from build123d import *

# Parameters (mm, degrees)
SKETCH_1_R               = 23.25
SKETCH_1_R_2             = 9
EXTRUDE_1_DEPTH          = 10
SKETCH_2_R               = 5
EXTRUDE_2_DEPTH          = 6
PATTERN_CIRCULAR_1_COUNT = 8
SKETCH_4_R               = 23.5
SKETCH_4_R_2             = 9
EXTRUDE_3_DEPTH          = 8.5


with BuildPart() as part:
    # 草图1 → 凸台-拉伸1 (new, symmetric)
    with BuildSketch(Plane(origin=(0, 0, 0), x_dir=(1, 0, 0), z_dir=(0, 1, 0))):
        with Locations(Location((0, 0, 0), (0, 0, 270))):
            Circle(SKETCH_1_R)
        with Locations(Location((0, 0, 0), (0, 0, 270))):
            Circle(SKETCH_1_R_2, mode=Mode.SUBTRACT)
    extrude(amount=EXTRUDE_1_DEPTH, both=True)

    # 草图2 → 凸台-拉伸2 (add)
    with BuildSketch(Plane(origin=(0, 10, 0), x_dir=(1, 0, 0), z_dir=(0, 1, 0))):
        with Locations(Location((16.25, 0, 0), (0, 0, 270))):
            Circle(SKETCH_2_R)
    extrude_2 = extrude(amount=EXTRUDE_2_DEPTH)

    # 阵列(圆周)1: 凸台-拉伸2 ×8 about axis
    pattern_circular_1_axis = Axis((0, 0, 0), (0, 1, 0))
    for i in range(1, PATTERN_CIRCULAR_1_COUNT):
        add(extrude_2.rotate(pattern_circular_1_axis, i * 360 / PATTERN_CIRCULAR_1_COUNT))

    # 草图4 → 凸台-拉伸3 (add, symmetric)
    with BuildSketch(Plane(origin=(0, 0, 0), x_dir=(1, 0, 0), z_dir=(0, 1, 0))):
        with Locations(Location((0, 0, 0), (0, 0, 270))):
            Circle(SKETCH_4_R)
        with Locations(Location((0, 0, 0), (0, 0, 270))):
            Circle(SKETCH_4_R_2, mode=Mode.SUBTRACT)
    extrude(amount=EXTRUDE_3_DEPTH, both=True)


solid = part.part
Geometry check sheet. Reference: the model listing, model coordinates, mm. A direction names the side the tool comes from. Give positions to 0.01 mm unless a question says otherwise; leave off trailing zeros. Loops run counter-clockwise (first coordinate to the right, second up) from the corner with the lowest first, then second, coordinate; pieces in that order, holes last.
(1) Section check B-B on x = 0. Record the cut outline in (y, z).
From the geometry:
outline: (-10, -23.25) - (-8.5, -23.25) - (-8.5, -23.5) - (8.5, -23.5) - (8.5, -23.25) - (10, -23.25) - (10, -21.25) - (16, -21.25) - (16, -11.25) - (10, -11.25) - (10, -9) - (-10, -9) - close; (-10, 9) - (10, 9) - (10, 11.25) - (16, 11.25) - (16, 21.25) - (10, 21.25) - (10, 23.25) - (8.5, 23.25) - (8.5, 23.5) - (-8.5, 23.5) - (-8.5, 23.25) - (-10, 23.25) - close
(2) Depth check by flat-ended pin: pin 1 Ø4 at (x, y) = (2.5, -1) entering from +Z; pin 2 Ø6 at (x, y) = (-18, 0.5) entering from -Z; pin 3 Ø1.5 at (y, z) = (-7, 16) entering from +X; pin 4 Ø11 at (x, z) = (0, 0) entering from +Y. Enter the tip coordinate at first touch or a pass-through.
From the geometry:
pin 1: stops at z = 23.49
pin 2: stops at z = -18.09
pin 3: stops at x = 17.88
pin 4: passes through
(3) Release check for a two-part mould opening along X. For faces 3 (the cylindrical face through (11.37, 12.96, -1.08)), 4 (the cylindrical face through (23.05, -9.24, -3.03)), 5 (the flat face through (0, 16, -16)) record: released by +X, released by -X, zero draft, split by the parting line, or undercut.
From the geometry:
face 3: undercut
face 4: split by the parting line
face 5: zero draft
(4) Section check A-A on z = 0. Record the cut outline in (x, y).
From the geometry:
outline: (-23.5, -8.5) - (-23.25, -8.5) - (-23.25, -10) - (-9, -10) - (-9, 10) - (-11.25, 10) - (-11.25, 16) - (-21.25, 16) - (-21.25, 10) - (-23.25, 10) - (-23.25, 8.5) - (-23.5, 8.5) - close; (9, -10) - (23.25, -10) - (23.25, -8.5) - (23.5, -8.5) - (23.5, 8.5) - (23.25, 8.5) - (23.25, 10) - (21.25, 10) - (21.25, 16) - (11.25, 16) - (11.25, 10) - (9, 10) - close
(5) Section check C-C on y = 11.75. Record the cut outline in (x, z), then the cut area to 3 significant figures.
From the geometry:
outline: circle Ø10 at (-16.25, 0); circle Ø10 at (-11.49, -11.49); circle Ø10 at (-11.49, 11.49); circle Ø10 at (0, -16.25); circle Ø10 at (0, 16.25); circle Ø10 at (11.49, -11.49); circle Ø10 at (11.49, 11.49); circle Ø10 at (16.25, 0)
area: 628 mm2
(6) Thickness scan on L1, parallel to X at y = 1.5, z = 0; L2, parallel to Y at x = 15, z = 6; L3, parallel to X at y = 14.75, z = 14.5. Record the ranges inside material, lowest first.
From the geometry:
L1: x = -23.5 to -9, 9 to 23.5
L2: y = -10 to 10
L3: x = -15.48 to -7.5, -4.68 to 4.68, 7.5 to 15.48
(7) Set-up check for faces 1 (the flat face through (16, 16, 0)), 2 (the cylindrical face through (1.08, 12.96, 11.37)): record each of +Z, -Z, +X, -X, +Y, -Y from which the full face is reachable in a straight line by a thin tool's end or side.
From the geometry:
face 1: +Z, -Z, +X, -X, +Y
face 2: +Y
(8) Section check D-D on x = -18. Record the cut outline in (y, z).
From the geometry:
outline: (-10, -14.72) - (-8.5, -14.72) - (-8.5, -15.11) - (8.5, -15.11) - (8.5, -14.72) - (10, -14.72) - (10, -4.68) - (16, -4.68) - (16, 4.68) - (10, 4.68) - (10, 14.72) - (8.5, 14.72) - (8.5, 15.11) - (-8.5, 15.11) - (-8.5, 14.72) - (-10, 14.72) - close
